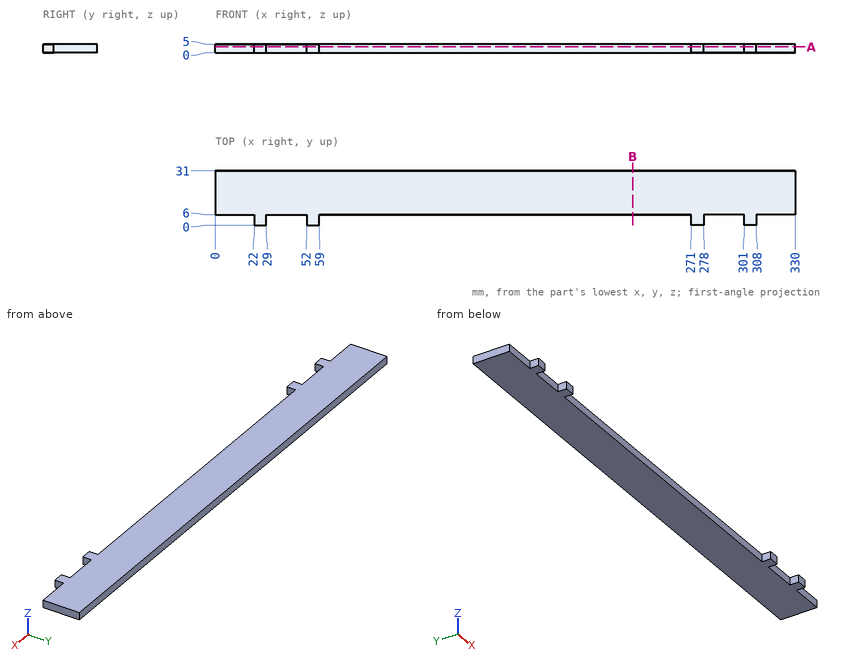
Geometry: see drawing. Coordinates: mm, zero at the bounding-box minimum. Give positions to 0.01 mm unless a question says otherwise; leave off trailing zeros. Order: outer loops, then holes, each group sorted by start corner. A loop starts at its lowest first (then second) coordinate and runs counter-clockwise, first axis right, second up.
Q1. Ray query, probe 1 along Y at (x, z) = (206, 4.8). Return the intervals inside material, ascending.
Checked values:
probe 1: y = 6 to 31
Q2. Contact query for flat-ended pins moving along their axis: pin 1 Ø2.5 at (x, z) = (285, 2) entering from -Y; pin 2 Ø1.5 at (y, z) = (3, 1.5) entering from -X; pin 3 Ø2.5 at (y, z) = (2, 2.5) entering from +X. Output: stop coordinate, or through.
Checked values:
pin 1: stops at y = 6
pin 2: stops at x = 22
pin 3: stops at x = 308
Q3. Section B-B on x = 237.5. Output: boundary loops of the cut face in (y, z).
Checked values:
outline: (6, 0) - (31, 0) - (31, 5) - (6, 5) - close
Q4. Section A-A on z = 3.3. Output: boundary loops of the cut face in (x, y).
Checked values:
outline: (0, 6) - (22, 6) - (22, 0) - (29, 0) - (29, 6) - (52, 6) - (52, 0) - (59, 0) - (59, 6) - (271, 6) - (271, 0) - (278, 0) - (278, 6) - (301, 6) - (301, 0) - (308, 0) - (308, 6) - (330, 6) - (330, 31) - (0, 31) - close
